Part print with two shaded views. Sizes in mm from the minimum x, y, z corner. A direction names the side the tool comes from. Give positions to 0.01 mm unless a question says otherwise; leave off trailing zeros. Order: outer loops, then holes, each group sorted by start corner. A loop starts at its lowest first (then second) coordinate and runs counter-clockwise, first axis right, second up. Notation, with made-up numbers: M -29,62.5 L -10,62.5 A22 cw -10,88.5 Z; hole C 81.25,38.25 d1. An arc over 180 degrees is marked long. Return JSON: item names as keys, results as strings.
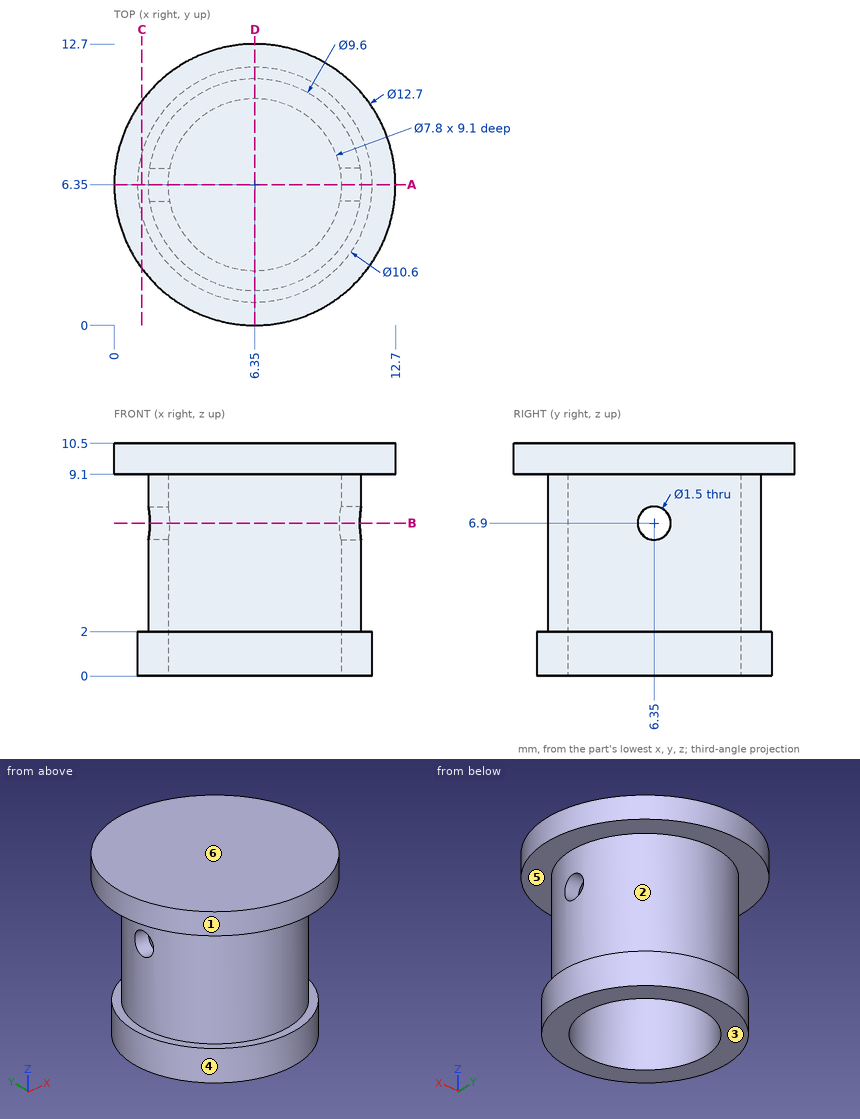
Q1. Band-saw the part on A-A (y = 6.35). Give the cut face in (x, z), then the cut area to 3 significant figures.
Established:
{"outline": "M 0,9.1 L 1.55,9.1 L 1.55,7.65 L 2.45,7.65 L 2.45,9.1 L 10.25,9.1 L 10.25,7.65 L 11.15,7.65 L 11.15,9.1 L 12.7,9.1 L 12.7,10.5 L 0,10.5 Z; M 1.05,0 L 2.45,0 L 2.45,6.15 L 1.55,6.15 L 1.55,2 L 1.05,2 Z; M 10.25,0 L 11.65,0 L 11.65,2 L 11.15,2 L 11.15,6.15 L 10.25,6.15 Z", "area": "33.5 mm²"}
Q2. Band-saw the part on D-D (x = 6.35). Give the cut face in (y, z).
Established:
{"outline": "M 0,9.1 L 1.55,9.1 L 1.55,2 L 1.05,2 L 1.05,0 L 2.45,0 L 2.45,9.1 L 10.25,9.1 L 10.25,0 L 11.65,0 L 11.65,2 L 11.15,2 L 11.15,9.1 L 12.7,9.1 L 12.7,10.5 L 0,10.5 Z"}
Q3. Two-plate mould, pull along Z, no slides. Class the marked faces 1, 2 and 3: +Z half, -Z half, draft (parallel to the pull), parting line (faces both ways), or undercut.
Established:
{"face 1": "draft", "face 2": "undercut", "face 3": "-Z half"}
Q4. 3-axis set-ups, long thin cutter, end or side, ignore diameter. For the marked faces 4, 5 and 6: which of +Z, -Z, +X, -X, +Y, -Y reach the whole face in a straight line?
Established:
{"face 4": "-Z", "face 5": "none", "face 6": "+Z, +X, -X, +Y, -Y"}
Q5. Probe line 1 along Z through (x, y) = (10.75, 3.5); line 2 along X through (y, z) = (6.35, 4); line 3 along Z through (x, y) = (10.45, 6.35). List the from-to ranges inside material, lowest first.
Established:
{"line 1": "z = 0 to 2, 9.1 to 10.5", "line 2": "x = 1.55 to 2.45, 10.25 to 11.15", "line 3": "z = 0 to 6.15, 7.65 to 10.5"}
Q6. Pin check, flat tips, straight feed: pin 1 (1 mm diameter, centred on y = 10.5, z = 6.5, fed in from -X); pin 2 (1.5 mm diameter, centred on x = 5, z = 6, fed in from +Y); pin 3 (1.7 mm diameter, centred on y = 6.35, z = 6.9, fed in from +X). Stop position of each tip, or through.
Established:
{"pin 1": "stops at x = 3.23", "pin 2": "stops at y = 11.11", "pin 3": "stops at x = 11.15"}
Q7. Band-saw the part on C-C (x = 1.25). Give the cut face in (y, z).
Established:
{"outline": "M 2.57,9.1 L 10.13,9.1 L 10.13,10.5 L 2.57,10.5 Z; M 4.91,0 L 7.79,0 L 7.79,2 L 4.91,2 Z"}
Q8. Band-saw the part on B-B (z = 6.9). Give the cut face in (x, y).
Established:
{"outline": "M 1.61,5.6 A4.8 ccw 11.09,5.6 L 10.18,5.6 A3.9 cw 2.52,5.6 Z; M 1.61,7.1 L 2.52,7.1 A3.9 cw 10.18,7.1 L 11.09,7.1 A4.8 ccw Z"}
